from build123d import *

# Parameters (mm, degrees)
SKETCH1_W           = 60
SKETCH1_H           = 7
BOSS_EXTRUDE1_DEPTH = 8.75
SKETCH2_W           = 26
SKETCH2_H           = 12.5
CUT_EXTRUDE1_DEPTH  = 8
SKETCH4_W           = 4
SKETCH4_H           = 1.1
CUT_EXTRUDE2_DEPTH  = 3.5
SKETCH5_W           = 8.2
SKETCH5_H           = 1.1
CUT_EXTRUDE4_DEPTH  = 0.65
SKETCH6_W           = 1.5
SKETCH6_H           = 1.1
CUT_EXTRUDE5_DEPTH  = 0.5
BOSS_EXTRUDE2_DEPTH = 2.5
SKETCH9_W           = 6
SKETCH9_H           = 2.5
BOSS_EXTRUDE4_DEPTH = 1.5
SKETCH10_W          = 25.5
SKETCH10_H          = 12.5
CUT_EXTRUDE6_DEPTH  = 5.5
CUT_EXTRUDE7_DEPTH  = 4
SKETCH12_W          = 60
SKETCH12_H          = 12.5
CUT_EXTRUDE8_DEPTH  = 0.25
FILLET1_R           = 4
FILLET2_R           = 5
FILLET3_R           = 1
CUT_EXTRUDE9_DEPTH  = 10
FILLET4_R           = 2
CHAMFER1_SIZE       = 0.75


with BuildPart() as part:
    # Sketch1 → Boss-Extrude1 (new body, symmetric)
    with BuildSketch(Plane.XY):
        with Locations((30, 3.5)):
            Rectangle(SKETCH1_W, SKETCH1_H)
    extrude(amount=BOSS_EXTRUDE1_DEPTH, both=True)

    # Sketch2 → Cut-Extrude1 (cut, through all)
    with BuildSketch(Plane(origin=(0, 7, 0), x_dir=(1, 0, 0), z_dir=(0, 1, 0))):
        with Locations((15, 0)):
            Rectangle(SKETCH2_W, SKETCH2_H)
    extrude(amount=-CUT_EXTRUDE1_DEPTH, mode=Mode.SUBTRACT)

    # Sketch3 → Cut-Revolve5 (revolve, cut)
    with BuildSketch(Plane.XY):
        Polygon((1.5, 5.9), (1.5, 5.15), (28, 5.15), (28, 3.9), (29.35, 3.9), (29.35, 1.8), (30, 1.8), (30, 3.9), (31.5, 3.9), (31.5, 5.9), align=None)
    revolve(axis=Axis((0, 5.9, 0), (1, 0, 0)), mode=Mode.SUBTRACT)

    # Sketch4 → Cut-Extrude2 (cut)
    with BuildSketch(Plane.ZY.offset(-28)):
        with Locations((0, 6.45)):
            Rectangle(SKETCH4_W, SKETCH4_H)
    extrude(amount=-CUT_EXTRUDE2_DEPTH, mode=Mode.SUBTRACT)

    # Sketch5 → Cut-Extrude4 (cut)
    with BuildSketch(Plane(origin=(29.35, 0, 0), x_dir=(0, 0, -1), z_dir=(1, 0, 0))):
        with Locations((0, 6.45)):
            Rectangle(SKETCH5_W, SKETCH5_H)
    extrude(amount=CUT_EXTRUDE4_DEPTH, mode=Mode.SUBTRACT)

    # Sketch6 → Cut-Extrude5 (cut)
    with BuildSketch(Plane(origin=(2, 0, 0), x_dir=(0, 0, -1), z_dir=(1, 0, 0))):
        with Locations((0, 6.45)):
            Rectangle(SKETCH6_W, SKETCH6_H)
    extrude(amount=-CUT_EXTRUDE5_DEPTH, mode=Mode.SUBTRACT)

    # Sketch7 → Boss-Extrude2 (add)
    with BuildSketch(Plane.XY.offset(8.75)):
        Polygon((54.5, 17.4625), (53.5, 17.098529766), (53.5, 12), (47.541232037, 7), (60, 7), (60, 12.9625), (63.5, 12.9625), (64.5, 13.326470234), (64.5, 17.098529766), (63.5, 17.4625), align=None)
    boss_extrude2 = extrude(amount=-BOSS_EXTRUDE2_DEPTH)

    # Sketch9 → Boss-Extrude4 (add)
    with BuildSketch(Plane.XZ):
        with Locations((3, 7.5)):
            Rectangle(SKETCH9_W, SKETCH9_H)
        with Locations((53, 7.5)):
            Rectangle(SKETCH9_W, SKETCH9_H)
    boss_extrude4 = extrude(amount=BOSS_EXTRUDE4_DEPTH)

    # Mirror1: Boss-Extrude2, Boss-Extrude4 across plane
    add(boss_extrude2.mirror(Plane.XY))
    add(boss_extrude4.mirror(Plane.XY))

    # Sketch10 → Cut-Extrude6 (cut)
    with BuildSketch(Plane(origin=(0, 7, 0), x_dir=(1, 0, 0), z_dir=(0, 1, 0))):
        with Locations((45.25, 0)):
            Rectangle(SKETCH10_W, SKETCH10_H)
    extrude(amount=-CUT_EXTRUDE6_DEPTH, mode=Mode.SUBTRACT)

    # Sketch11 → Cut-Extrude7 (cut, through all)
    with BuildSketch(Plane(origin=(0, 1.5, 0), x_dir=(1, 0, 0), z_dir=(0, 1, 0))):
        with BuildLine():
            Line((52.35, -2.38125), (48.35, -2.38125))
            ThreePointArc((48.35, -2.38125), (45.96875, 0), (48.35, 2.38125))
            Line((48.35, 2.38125), (52.35, 2.38125))
            ThreePointArc((52.35, 2.38125), (54.73125, 0), (52.35, -2.38125))
        make_face()
    extrude(amount=-CUT_EXTRUDE7_DEPTH, mode=Mode.SUBTRACT)

    # Sketch12 → Cut-Extrude8 (cut)
    with BuildSketch(Plane.XZ):
        with Locations((30, 0)):
            Rectangle(SKETCH12_W, SKETCH12_H)
    extrude(amount=-CUT_EXTRUDE8_DEPTH, mode=Mode.SUBTRACT)

    # Fillet1
    fillet1_edges = [part.edges().sort_by_distance(p)[0] for p in [
        (59, 7, -6.25),
        (59, 7, 6.25),
    ]]
    fillet(fillet1_edges, radius=FILLET1_R)

    # Fillet2
    fillet2_edges = [part.edges().sort_by_distance(p)[0] for p in [
        (47.541232037, 7, 7.5),
        (47.541232037, 7, -7.5),
    ]]
    fillet(fillet2_edges, radius=FILLET2_R)

    # Fillet3
    fillet3_edges = [part.edges().sort_by_distance(p)[0] for p in [
        (58, 4.25, -6.25),
        (58, 4.25, 6.25),
        (32.5, 4.25, 6.25),
        (32.5, 4.25, -6.25),
        (28, 3.625, 6.25),
        (2, 3.625, 6.25),
        (28, 3.625, -6.25),
        (2, 3.625, -6.25),
    ]]
    fillet(fillet3_edges, radius=FILLET3_R)

    # Sketch13 → Cut-Extrude9 (cut)
    with BuildSketch(Plane(origin=(0, 0, -8.75), x_dir=(-1, 0, 0), z_dir=(0, 0, -1))):
        with BuildLine():
            Line((-2, 7), (-2, 5.9))
            ThreePointArc((-2, 5.9), (-2.585786438, 4.485786438), (-4, 3.9))
            Line((-4, 3.9), (-7, 3.9))
            ThreePointArc((-7, 3.9), (-8.414213562, 4.485786438), (-9, 5.9))
            Line((-9, 5.9), (-9, 7))
            Line((-9, 7), (-2, 7))
        make_face()
    extrude(amount=-CUT_EXTRUDE9_DEPTH, mode=Mode.SUBTRACT)

    # Fillet4
    fillet4_edges = [part.edges().sort_by_distance(p)[0] for p in [
        (53.5, 12, -7.5),
        (53.5, 12, 7.5),
    ]]
    fillet(fillet4_edges, radius=FILLET4_R)

    # Chamfer1
    chamfer1_edges = [part.edges().sort_by_distance(p)[0] for p in [
        (28, 3.9, 0),
        (28, 6.45, 2),
        (28, 6.45, -2),
    ]]
    chamfer(chamfer1_edges, length=CHAMFER1_SIZE)


solid = part.part
Build history of the part. All positions in model axes, mm. A direction names the side the tool comes from. Round coordinates to 2 decimals unless told otherwise and drop trailing zeros. Write each loop counter-clockwise with the first axis right and the second up, starting at its lowest first coordinate (ties: lowest second). Pieces come first, ordered by that corner, then holes. Notation, with made-up numbers: (-24.5, -32) -> (-16.5, -32) arc R26 ccw to (-16.5, 3) -> close; hole circle Ø3 at (83, 39). An arc over 180 degrees is marked (long way). Use one line per item in the form item = value.
Q1. Band-saw the part on C-C, the plane x = 17.5. Write the cut outline in (y, z), then the cut area to 3 significant figures.
Conclusion:
outline = (0, -8.75) -> (7, -8.75) -> (7, -6.25) -> (0, -6.25) -> close; (0, 6.25) -> (7, 6.25) -> (7, 8.75) -> (0, 8.75) -> close
area = 35.0 mm²
Q2. Tool access for faces 1 (the cylindrical face through (45.97, 0.88, 0.05)), 2 (the flat face through (6, -1, 7)), 3 (the cylindrical face through (30.8, 3.9, 0)): list every direction of +Z, -Z, +X, -X, +Y, -Y with a clear straight run to the whole face (end or side of a thin tool).
Conclusion:
face_1 = +Y, -Y
face_2 = +Z, -Z, -Y
face_3 = +Y
Q3. Band-saw the part on A-A, the plane z = 0. Write the cut outline in (x, y), then the cut area to 3 significant figures.
Conclusion:
outline = (0, 0.25) -> (2, 0.25) -> (2, 5.15) -> (1.5, 5.15) -> (1.5, 7) -> (0, 7) -> close; (28, 0.25) -> (45.97, 0.25) -> (45.97, 1.5) -> (32.5, 1.5) -> (32.5, 7) -> (31.5, 7) -> (31.5, 3.9) -> (30, 3.9) -> (30, 1.8) -> (29.35, 1.8) -> (29.35, 3.9) -> (28.75, 3.9) -> (28, 3.15) -> close; (54.73, 0.25) -> (60, 0.25) -> (60, 7) -> (58, 7) -> (58, 1.5) -> (54.73, 1.5) -> close
area = 64.9 mm²
Q4. Band-saw the part on D-D, the plane z = -7.5. Write the cut outline in (x, y).
Conclusion:
outline = (0, -1.5) -> (6, -1.5) -> (6, 0) -> (50, 0) -> (50, -1.5) -> (56, -1.5) -> (56, 0) -> (60, 0) -> (60, 12.96) -> (63.5, 12.96) -> (64.5, 13.33) -> (64.5, 17.1) -> (63.5, 17.46) -> (54.5, 17.46) -> (53.5, 17.1) -> (53.5, 12.93) arc R2 cw to (52.79, 11.4) -> (48.94, 8.17) arc R5 cw to (45.72, 7) -> (9, 7) -> (9, 5.9) arc R2 cw to (7, 3.9) -> (4, 3.9) arc R2 cw to (2, 5.9) -> (2, 7) -> (0, 7) -> close
Q5. Two-plate mould, pull along Z, no slides. Class faces 4 (the flat face through (37, 5, -8.75)), 5 (the flat face through (45, 1.5, 0)), 6 (the flat face through (50, -1, 7)): released by +Z, released by -Z, zero draft, split by the parting line, or undercut.
Conclusion:
face_4 = released by -Z
face_5 = undercut
face_6 = zero draft
Q6. Band-saw the part on B-B, the plane y = 15.25. Write the cut outline in (x, z).
Conclusion:
outline = (53.5, -8.75) -> (64.5, -8.75) -> (64.5, -6.25) -> (53.5, -6.25) -> close; (53.5, 6.25) -> (64.5, 6.25) -> (64.5, 8.75) -> (53.5, 8.75) -> close
Q7. Drill centre lines: L1, parallel to Z at x = 56, y = 12; L2, parallel to X at y = 3.75, z = 3; L3, parallel to X at y = 5.25, z = 6. Where is each one in solid material? Low to high.
Conclusion:
L1 = -8.75 to -6.25, 6.25 to 8.75
L2 = 0 to 2, 28 to 29.35, 30 to 32.5, 58 to 60
L3 = 0 to 2.34, 27.66 to 32.84, 57.66 to 60
Q8. Drop flat-ended pins along their axis: P1, Ø3, axis at x = 61, z = 8, coming from the -Y side; P2, Ø4, axis at x = 52.5, y = 14, coming from the -Z side; P3, Ø0.8, axis at y = 14, z = 7.5, coming from the -X side; P4, Ø1.2, axis at x = 61.5, z = -7.5, coming from the -Y side. Give the stop position or say it passes through.
Conclusion:
P1 = 0
P2 = -8.75
P3 = 53.5
P4 = 12.96
